```python
from build123d import *

# Parameters (mm, degrees)
SKETCH1_W           = 9
SKETCH1_H           = 45
SKETCH1_R           = 1.63195
BOSS_EXTRUDE1_DEPTH = 40
SKETCH1_3_R         = 1.63195
CUT_EXTRUDE1_DEPTH  = 10
SKETCH2_W           = 40
SKETCH2_H           = 3
CUT_EXTRUDE2_DEPTH  = 6
CUT_EXTRUDE3_DEPTH  = 9
CUT_EXTRUDE4_DEPTH  = 6
CHAMFER2_SIZE       = 4
SKETCH6_R           = 2.0193
CUT_EXTRUDE5_DEPTH  = 6
SKETCH7_W           = 3
SKETCH7_H           = 30
BOSS_EXTRUDE3_DEPTH = 9.52
CHAMFER3_SIZE       = 4
FILLET1_R           = 2
SKETCH8_W           = 73.917674983
SKETCH8_H           = 61.996597993
CUT_EXTRUDE6_DEPTH  = 9


with BuildPart() as part:
    # Sketch1 → Boss-Extrude1 (new body)
    # profile 1 of 3: a face of its own
    with BuildSketch(Plane.XY):
        with Locations((4.5, 22.5)):
            Rectangle(SKETCH1_W, SKETCH1_H)
        with Locations((6, 13)):
            Circle(SKETCH1_R, mode=Mode.SUBTRACT)
        with Locations((6, 25)):
            Circle(SKETCH1_R, mode=Mode.SUBTRACT)
    # profile 2 of 3: a face of its own
    with BuildSketch(Plane.XY):
        with Locations((6, 25)):
            Circle(SKETCH1_R)
    # profile 3 of 3: a face of its own
    with BuildSketch(Plane.XY):
        with Locations((6, 13)):
            Circle(SKETCH1_R)
    extrude(amount=BOSS_EXTRUDE1_DEPTH)

    # Sketch1<3> → Cut-Extrude1 (cut)
    with BuildSketch(Plane.XY):
        with Locations((6, 25)):
            Circle(SKETCH1_3_R)
        with Locations((6, 13)):
            Circle(SKETCH1_3_R)
    extrude(amount=CUT_EXTRUDE1_DEPTH, mode=Mode.SUBTRACT)

    # Sketch2 → Cut-Extrude2 (cut)
    with BuildSketch(Plane(origin=(9, 0, 0), x_dir=(0, 0, -1), z_dir=(1, 0, 0))):
        with Locations((-20, 6.2)):
            Rectangle(SKETCH2_W, SKETCH2_H)
    extrude(amount=-CUT_EXTRUDE2_DEPTH, mode=Mode.SUBTRACT)

    # Sketch3 → Cut-Extrude3 (cut)
    with BuildSketch(Plane(origin=(9, 0, 0), x_dir=(0, 0, -1), z_dir=(1, 0, 0))):
        Polygon((-20, 45), (-40, 15), (-48.379363257, 51.913157268), align=None)
    extrude(amount=-CUT_EXTRUDE3_DEPTH, mode=Mode.SUBTRACT)

    # Sketch5 → Cut-Extrude4 (cut)
    with BuildSketch(Plane.ZY):
        Polygon((20, 45), (10, 45), (13.204776383, 21.55213026), (40, 12), (40, 15), align=None)
    extrude(amount=-CUT_EXTRUDE4_DEPTH, mode=Mode.SUBTRACT)

    # Chamfer2
    chamfer2_edges = [part.edges().sort_by_distance(p)[0] for p in [
        (0, 33.27606513, 11.602388192),
        (0, 16.77606513, 26.602388192),
    ]]
    chamfer(chamfer2_edges, length=CHAMFER2_SIZE)

    # Sketch6 → Cut-Extrude5 (cut)
    with BuildSketch(Plane.XZ):
        with Locations(Location((5.5, 35, 0), (0, 0, 270))):
            Circle(SKETCH6_R)
        with Locations(Location((5.5, 20, 0), (0, 0, 270))):
            Circle(SKETCH6_R)
    extrude(amount=-CUT_EXTRUDE5_DEPTH, mode=Mode.SUBTRACT)

    # Sketch7 → Boss-Extrude3 (add)
    with BuildSketch(Plane(origin=(0, 0, 0), x_dir=(-1, 0, 0), z_dir=(0, 0, -1))):
        with Locations((-1.5, 30)):
            Rectangle(SKETCH7_W, SKETCH7_H)
    extrude(amount=BOSS_EXTRUDE3_DEPTH)

    # Chamfer3
    chamfer3_edges = [part.edges().sort_by_distance(p)[0] for p in [
        (1.5, 15, 0),
    ]]
    chamfer(chamfer3_edges, length=CHAMFER3_SIZE)

    # Fillet1
    fillet1_edges = [part.edges().sort_by_distance(p)[0] for p in [
        (1.5, 45, -9.52),
        (1.5, 15, -9.52),
    ]]
    fillet(fillet1_edges, radius=FILLET1_R)

    # Mirror1: part across plane


with BuildPart() as part_1:
    add(part.part)
    add(part.part.mirror(Plane(origin=(9, 0, 40), x_dir=(0, 0, 1), z_dir=(-1, 0, 0))))

    # Sketch8 → Cut-Extrude6 (cut)
    with BuildSketch(Plane(origin=(0, 0, 0), x_dir=(0, 0, -1), z_dir=(1, 0, 0))):
        with Locations((-12.663539667, 19.880173389)):
            Rectangle(SKETCH8_W, SKETCH8_H)
    extrude(amount=CUT_EXTRUDE6_DEPTH, mode=Mode.SUBTRACT)


solid = part_1.part
```
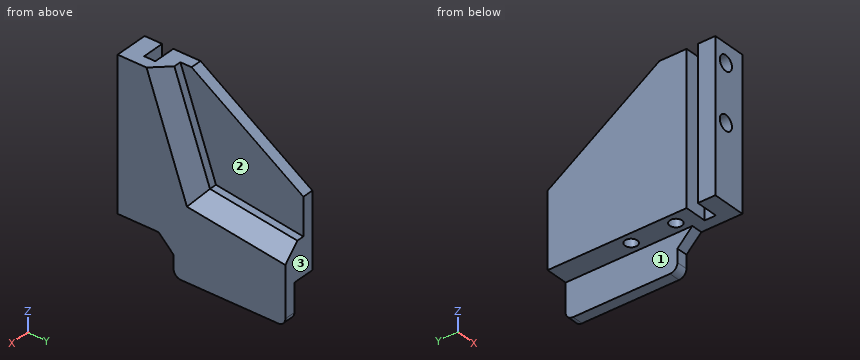
Verification items for the finished model (mm, model axes). Face numbers are marked on the shaded views. A direction names the side the tool comes from. Give positions to 0.01 mm unless a question says otherwise; leave off trailing zeros. Loops run counter-clockwise (first coordinate to the right, second up) from the corner with the lowest first, then second, coordinate; pieces in that order, holes last.
1. Section check D-D, the plane y = 13. Enter the section's corners in (x, z).
2. Section check B-B, the plane z = 35. Enter the section's corners in (x, y).
3. Thickness scan on line 1 (Z direction, x = 12.5, y = 1.8); line 2 (Y direction, x = 12, z = 5); line 3 (Y direction, x = 13.75, z = 5). Record the ranges inside material, lowest first.
4. Section check A-A, the plane z = 5. Enter the section's corners in (x, y).
5. Set-up check for the marked faces 1, 2 and 3: record each of +Z, -Z, +X, -X, +Y, -Y from which the full face is reachable in a straight line by a thin tool's end or side.
6. Section check C-C, the plane x = 17.25. Enter the section's corners in (y, z).
7. Go/stop test with flat-tipped pins: pin 1 Ø0.9 at (x, z) = (16, -6.5) entering from -Y; pin 2 Ø5 at (x, z) = (12.5, 25.5) entering from +Y; pin 3 Ø3 at (x, z) = (12.5, 35) entering from -Y. Record where each tip stops, or that it passes through.
Geometry says:
1. outline: (9, 0) - (10.37, 0) - (10.37, 10) - (13.63, 10) - (13.63, 0) - (15, 0) - (15, -2) - (18, -2) - (18, 25.28) - (14, 37.19) - (12, 37.19) - (12, 40) - (9, 40) - close
2. outline: (9, 0) - (10.48, 0) - (10.48, 4.7) - (9, 4.7) - close; (9, 7.7) - (15, 7.7) - (15, 4.7) - (14.52, 4.7) - (14.52, 0) - (18, 0) - (18, 9.54) - (14, 13.78) - (12, 13.78) - (12, 22.5) - (9, 22.5) - close
3. line 1: z = 0 to 17.98, 22.02 to 32.98, 37.02 to 40
3. line 2: y = 0 to 4.7, 7.7 to 11.37, 14.63 to 23.37, 26.63 to 45
3. line 3: y = 0 to 4.7, 7.7 to 45
4. outline: (9, 0) - (18, 0) - (18, 45) - (9, 45) - (9, 7.7) - (15, 7.7) - (15, 4.7) - (9, 4.7) - close; hole circle Ø3.26 at (12, 13); hole circle Ø3.26 at (12, 25)
5. face 1: -Z, -X, +Y, -Y
5. face 2: +Z, +X, +Y
5. face 3: +Z, -Z, +X, -X, +Y
6. outline: (0, 0) - (11, 0) - (15, -4) - (15, -7.52) arc R2 ccw to (17, -9.52) - (43, -9.52) arc R2 ccw to (45, -7.52) - (45, 6.72) - (19.15, 10.25) - (8.55, 40) - (0, 40) - close
7. pin 1: stops at y = 15
7. pin 2: stops at y = 40.42
7. pin 3: stops at y = 7.7
